Job drawing, mm, ordinate dimensions from the low corner. One solid piece. A direction names the side the tool comes from. Give positions to 0.01 mm unless a question says otherwise; leave off trailing zeros. Order: outer loops, then holes, each group sorted by start corner. A loop starts at its lowest first (then second) coordinate and runs counter-clockwise, first axis right, second up.
Item 1: Band-saw the part on A-A on y = 27.07. Give the cut face in (x, z).
Item 2: Flat gauge pins, fed straight in: P1, Ø2, axis at x = 34.5, z = 14.5, coming from the +Y side; P2, Ø11.5, axis at y = 20.5, z = 15, coming from the +X side; P3, Ø6, axis at x = 7.5, z = 13.5, coming from the +Y side; P4, Ø7, axis at y = 21, z = 12.5, coming from the -X side. Where does each tip first touch, or does it go through?
Item 3: Band-saw the part on B-B on z = 21. Give the cut face in (x, y).
Item 4: Wall check: L1, parallel to X at y = 3, z = 8; L2, parallel to X at y = 30, z = 20.75; L3, parallel to Y at x = 17, z = 5. Give the ranges that are in metal, low to high.
Item 5: Band-saw the part on D-D on y = 2. Give the cut face in (x, z), plus the area to 3 significant figures.
Item 6: Which spindle directions (+Z, -Z, +X, -X, +Y, -Y) get a long thin tool onto all of the face, cutting with end or side? Do the marked faces 1 and 2. Say none if no direction does.
Item 7: Band-saw the part on C-C on x = 38.5. Give the cut face in (y, z) (3 decimals), plus the area to 3 significant figures.
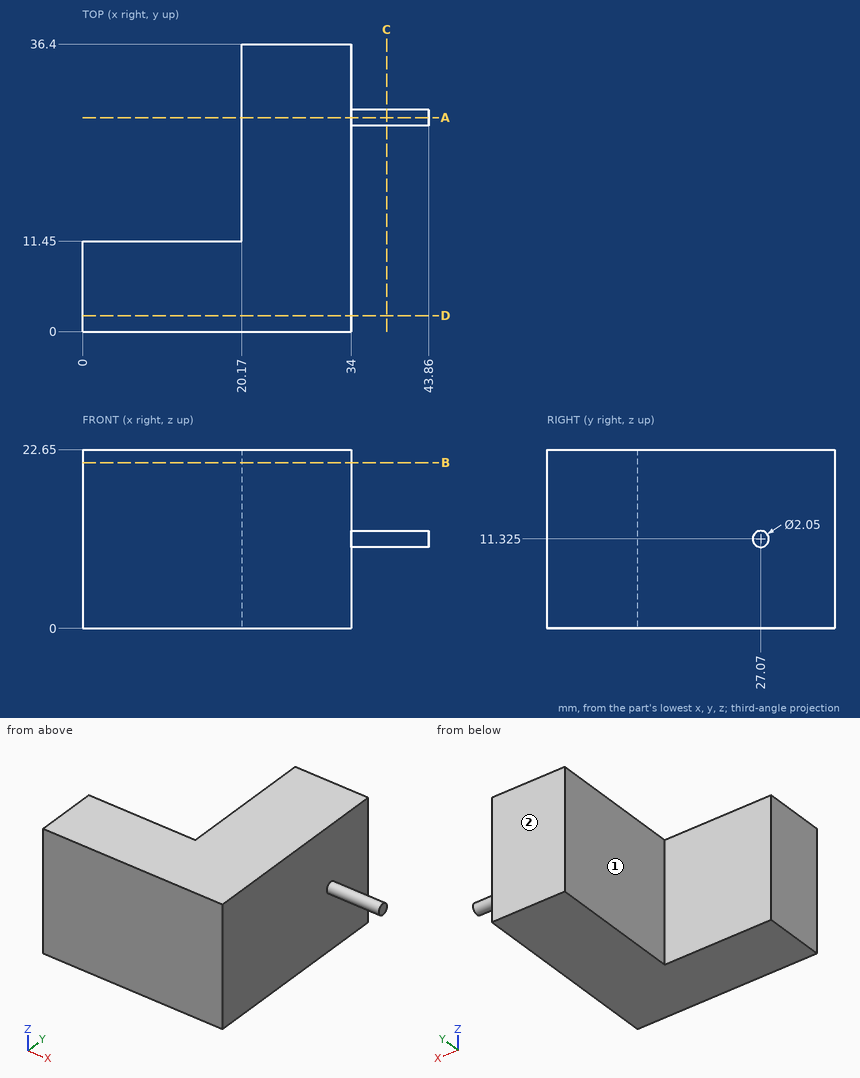
The answers:
1. outline: (20.17, 0) - (34, 0) - (34, 10.3) - (43.86, 10.3) - (43.86, 12.35) - (34, 12.35) - (34, 22.65) - (20.17, 22.65) - close
2. P1: stops at y = 36.4
2. P2: stops at x = 34
2. P3: stops at y = 11.45
2. P4: stops at x = 20.17
3. outline: (0, 0) - (34, 0) - (34, 36.4) - (20.17, 36.4) - (20.17, 11.45) - (0, 11.45) - close
4. L1: x = 0 to 34
4. L2: x = 20.17 to 34
4. L3: y = 0 to 11.45
5. outline: (0, 0) - (34, 0) - (34, 22.65) - (0, 22.65) - close
5. area: 770 mm2
6. face 1: +Z, -Z, -X, +Y
6. face 2: +Z, -Z, +X, -X, +Y
7. outline: circle Ø2.05 at (27.07, 11.325)
7. area: 3.30 mm2
